The drawing under review shows one solid part. Ordinate dimensions are in mm from its lowest x, y, z. Coordinates: 2 decimals unless noted, no trailing zeros. Loops run counter-clockwise (first coordinate to the right, second up) from the corner with the lowest first, then second, coordinate; pieces in that order, holes last.
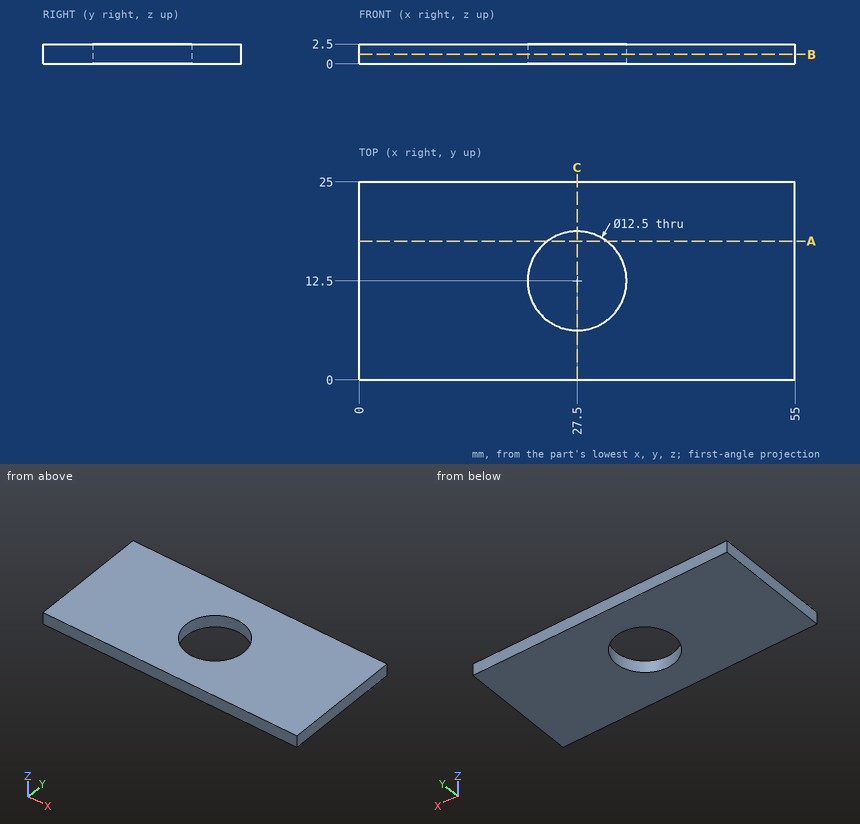
Q1. Take a section at C-C, the plane x = 27.5. Write out the cut boundary in (y, z), then the cut area to 4 significant figures.
Q2. For line 1 (Y direction, x = 27.5, z = 1.05); line 2 (X direction, y = 17, z = 1.6); line 3 (Y direction, x = 30, z = 1), list the stretches that pass through material, from the lowest coordinate up.
Q3. Take a section at A-A, the plane y = 17.5. Write out the cut boundary in (x, z), then the cut area to 3 significant figures.
Q4. Take a section at B-B, the plane z = 1.2. Write out the cut boundary in (x, y).
Entries:
1. outline: (0, 0) - (6.25, 0) - (6.25, 2.5) - (0, 2.5) - close; (18.75, 0) - (25, 0) - (25, 2.5) - (18.75, 2.5) - close
1. area: 31.25 mm2
2. line 1: y = 0 to 6.25, 18.75 to 25
2. line 2: x = 0 to 23.16, 31.84 to 55
2. line 3: y = 0 to 6.77, 18.23 to 25
3. outline: (0, 0) - (23.75, 0) - (23.75, 2.5) - (0, 2.5) - close; (31.25, 0) - (55, 0) - (55, 2.5) - (31.25, 2.5) - close
3. area: 119 mm2
4. outline: (0, 0) - (55, 0) - (55, 25) - (0, 25) - close; hole circle Ø12.5 at (27.5, 12.5)
